Autodesk Inventor part; units mm, degrees
ref_plane "Work Plane2" through (0, 0, -17.465) normal (0, 0, 1) x (1, 0, 0)
ref_plane "Work Plane3" through (0, 4.765, 0) normal (0, -1, 0) x (1, 0, 0)
ref_plane "YZ Plane" through (0, 0, 0) normal (1, 0, 0) x (0, 1, 0)
sketch "Sketch1" plane through (0, 0, 0) normal (0, 1, 0) x (-1, 0, 0)
  line L0 (0, 0) -> (-4.75, 0)
  line L1 (-4.75, 0) -> (-4.75, -34.93)
  line L2 (-4.75, -34.93) -> (0, -34.93)
  line L3 (0, -34.93) -> (0, 0)
  line L4 (-4.75, 0) -> (-23.8, 0)
  line L5 (-23.8, 0) -> (-23.8, -4.565)
  line L6 (-23.8, -4.565) -> (-4.75, -4.565)
  line L7 (-4.75, -4.565) -> (-4.75, 0)
  line L8 (-4.75, -12.7) -> (-23.8, -12.7)
  line L9 (-23.8, -12.7) -> (-23.8, -22.23)
  line L10 (-23.8, -22.23) -> (-4.75, -22.23)
  line L11 (-4.75, -22.23) -> (-4.75, -12.7)
  line L12 (-4.75, -34.93) -> (-23.8, -34.93)
  line L13 (-23.8, -34.93) -> (-23.8, -30.365)
  line L14 (-23.8, -30.365) -> (-4.75, -30.365)
  line L15 (-4.75, -30.365) -> (-4.75, -34.93)
  line L16 (0, -17.465) -> (-23.9272, -17.465) construction
  point P0 (-23.8, -17.465)
  dimension "d0" = 34.93
  dimension "d1" = 9.53
  dimension "d2" = 25.8
  dimension "d3" = 12.9
  dimension "d4" = 19.05
  dimension "d5" = 23.8
extrude "Extrusion1" add sketch "Sketch1" along normal blind 9.53
ref_plane "Work Plane2" through (0, 0, -17.465) normal (0, 0, 1) x (1, 0, 0)
ref_plane "Work Plane3" through (0, 4.765, 0) normal (0, -1, 0) x (1, 0, 0)
equation "\"d3\" = 0.5 * d2"
properties part number "TSC_EL375" material "Iron, Gray"
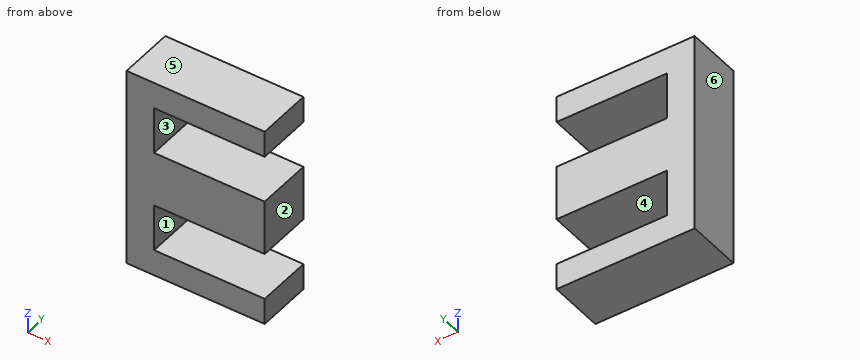
Read the model definition and answer for the solid it produces. Units are mm, in the model's axes. Face numbers are marked on the shaded views. A direction names the side the tool comes from. Coordinates: 2 decimals unless noted, no trailing zeros. Loops run counter-clockwise (first coordinate to the right, second up) from the corner with the lowest first, then second, coordinate; pieces in that order, holes last. Notation, with made-up numbers: (-40, 55.25) -> (-36, 55.25) arc R15 cw to (-36, 80.25) -> close; hole circle Ø4 at (-5, -9.75). An arc over 180 degrees is marked (long way). Answer in a Markdown table with one row per item.
Item 1: Straight lines are drawn through the part: line 1 along Z through (x, y) = (11, 1.75) (3 decimals); line 2 along X through (y, z) = (4.25, -28). For each, find the intervals that lie inside material, in ascending order. Write a range as [from, to].
Returned:
| item | result |
|---|---|
| line 1 | z = [-34.93, -30.365], [-22.23, -12.7], [-4.565, 0] |
| line 2 | x = [0, 4.75] |
Item 2: For a pull along Z with two mould halves and no side action, classify the marked faces 3, 4, 5 and 6 as released by +Z, released by -Z, zero draft, split by the parting line, or undercut.
Returned:
| item | result |
|---|---|
| face 3 | undercut |
| face 4 | undercut |
| face 5 | released by +Z |
| face 6 | zero draft |
Item 3: A cutting plane is placed at C-C on z = -30. Determine the outline of the cut face in (x, y).
Returned:
| item | result |
|---|---|
| outline | (0, 0) -> (4.75, 0) -> (4.75, 9.53) -> (0, 9.53) -> close |
Item 4: A cutting plane is placed at B-B on y = 5.25. Determine the outline of the cut face in (x, z) (3 decimals), plus the area to 3 significant figures.
Returned:
| item | result |
|---|---|
| outline | (0, -34.93) -> (23.8, -34.93) -> (23.8, -30.365) -> (4.75, -30.365) -> (4.75, -22.23) -> (23.8, -22.23) -> (23.8, -12.7) -> (4.75, -12.7) -> (4.75, -4.565) -> (23.8, -4.565) -> (23.8, 0) -> (0, 0) -> close |
| area | 521 mm^2 |
Item 5: For the marked faces 1 and 2, determine the directions among +Z, -Z, +X, -X, +Y, -Y from which every point of the face is accessible in a straight line to the end or side of a thin tool.
Returned:
| item | result |
|---|---|
| face 1 | +X, +Y, -Y |
| face 2 | +Z, -Z, +X, +Y, -Y |
Item 6: A cutting plane is placed at A-A on x = 13. Determine the outline of the cut face in (y, z) (3 decimals).
Returned:
| item | result |
|---|---|
| outline | (0, -34.93) -> (9.53, -34.93) -> (9.53, -30.365) -> (0, -30.365) -> close; (0, -22.23) -> (9.53, -22.23) -> (9.53, -12.7) -> (0, -12.7) -> close; (0, -4.565) -> (9.53, -4.565) -> (9.53, 0) -> (0, 0) -> close |
